The figure shows three views and two pictorial views of one solid part (mm, origin at its lowest corner). Answer the questions. A direction names the side the tool comes from. Give positions to 0.01 mm unless a question says otherwise; leave off trailing zeros. Loops run counter-clockwise (first coordinate to the right, second up) from the corner with the lowest first, then second, coordinate; pieces in that order, holes last. Notation, with made-up numbers: (58, 7.5) - (87, 7.5) arc R22 ccw to (87, 44.5) - close; hole circle Ø11 at (67, 41). An arc over 180 degrees is marked (long way). One line per question, with ' | ' between items.
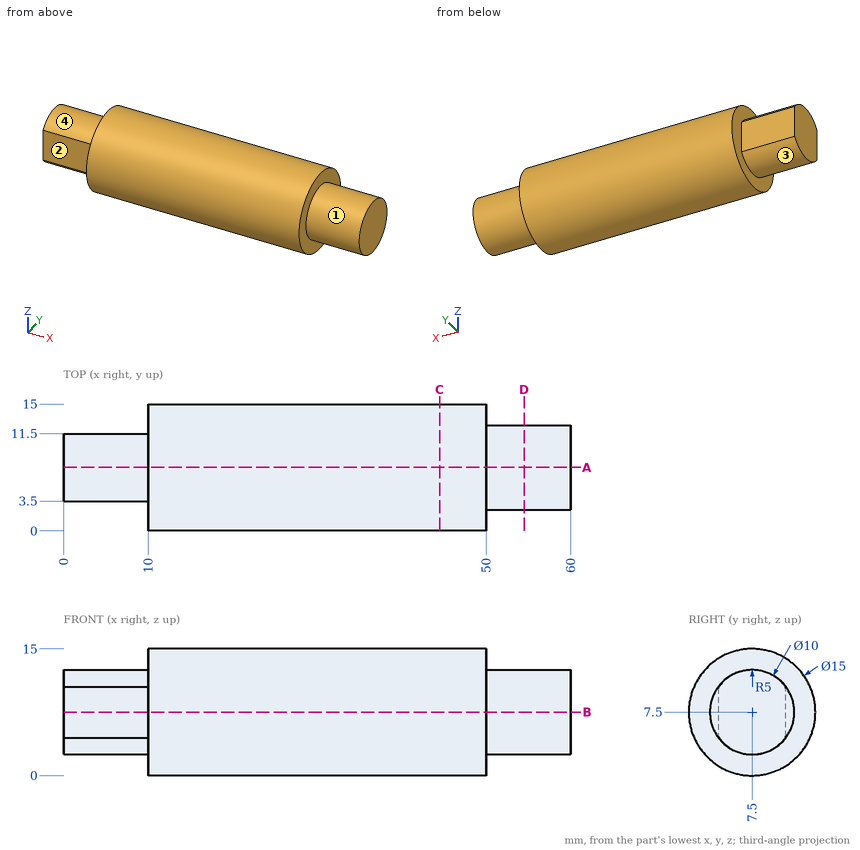
1. Which of the six approach directions +Z, -Z, +X, -X, +Y, -Y give full straight-line access (tool end or side, diameter ignored) to the marked faces 1, 2, 3 and 4?
Evaluation:
face 1: +X | face 2: +Z, -Z, -X, -Y | face 3: -Z, -X | face 4: +Z, -X
2. Find section A-A on y = 7.5. Write down the section's boundary in (x, z).
Evaluation:
outline: (0, 2.5) - (10, 2.5) - (10, 0) - (50, 0) - (50, 2.5) - (60, 2.5) - (60, 12.5) - (50, 12.5) - (50, 15) - (10, 15) - (10, 12.5) - (0, 12.5) - close
3. Consider L1, parallel to X at y = 13.25, z = 5; L2, parallel to Z at x = 38, y = 7.75; L3, parallel to Z at x = 57, y = 7.25. Determine where each line is inside the solid, lowest interval first.
Evaluation:
L1: 10 to 50 | L2: 0 to 15 | L3: 2.51 to 12.49
4. Find section C-C on x = 44.5. Write down the section's boundary in (y, z), then the cut area to 3 significant figures.
Evaluation:
outline: circle Ø15 at (7.5, 7.5) | area: 177 mm2
5. Flat-ended cylindrical pins translate along their axes: pin 1 (3 mm diameter, centred on x = 24, y = 13.5, fed in from +Z); pin 2 (5 mm diameter, centred on x = 3.5, z = 7, fed in from +Y); pin 3 (6 mm diameter, centred on x = 35, z = 4, fed in from +Y). Find the tip coordinate at first contact, or state that the pin passes through.
Evaluation:
pin 1: z = 13.5 | pin 2: y = 11.5 | pin 3: y = 14.98
6. Find section D-D on x = 54.5. Write down the section's boundary in (y, z).
Evaluation:
outline: circle Ø10 at (7.5, 7.5)
7. Find section B-B on z = 7.5. Write down the section's boundary in (x, y), then the cut area to 3 significant figures.
Evaluation:
outline: (0, 3.5) - (10, 3.5) - (10, 0) - (50, 0) - (50, 2.5) - (60, 2.5) - (60, 12.5) - (50, 12.5) - (50, 15) - (10, 15) - (10, 11.5) - (0, 11.5) - close | area: 780 mm2
